from build123d import *

# Parameters (mm, degrees)
BOSS_EXTRUDE1_DEPTH = 10
BOSS_EXTRUDE2_DEPTH = 10
FILLET1_R           = 1


with BuildPart() as part:
    # Sketch1 → Boss-Extrude1 (new body)
    with BuildSketch(Plane(origin=(0, 0, 0), x_dir=(1, 0, 0), z_dir=(0, 1, 0))):
        Polygon((0, 0), (2, 0.535898385), (2, 23.5), (0, 23.5), align=None)
    extrude(amount=BOSS_EXTRUDE1_DEPTH)

    # Sketch3 → Boss-Extrude2 (add)
    with BuildSketch(Plane.XZ):
        Polygon((0, 0), (115.911099155, -31.058285412), (115.285791267, -32.958019616), (0, -2), align=None)
    extrude(amount=-BOSS_EXTRUDE2_DEPTH)

    # Fillet1
    fillet1_edges = [part.edges().sort_by_distance(p)[0] for p in [
        (2, 5, -2.537065657),
        (0, 5, 0),
    ]]
    fillet(fillet1_edges, radius=FILLET1_R)


solid = part.part
Geometry check sheet. Reference: the model listing, model coordinates, mm. A direction names the side the tool comes from. Coordinates: 2 decimals unless noted, no trailing zeros. Order: outer loops, then holes, each group sorted by start corner. A loop starts at its lowest first (then second) coordinate and runs counter-clockwise, first axis right, second up. Notation, with made-up numbers: (68, 14) -> (123, 14) arc R35 cw to (123, 51) -> close; hole circle Ø10 at (51, -10). An arc over 180 degrees is marked (long way). Use a Markdown table: item, result. Add a question column.
1. Go/stop test with flat-tipped pins: pin 1 Ø5 at (x, y) = (69, 8.5) entering from -Z; pin 2 Ø0.6 at (x, y) = (1, 2.5) entering from -Z; pin 3 Ø1 at (x, y) = (26.5, 4.5) entering from -Z. Record where each tip stops, or that it passes through.
2. Cross-section at C-C (z = -10). Enter the section's corners in (x, y), and give its area (3 significant figures).
3. Set-up check for faces 1 (the face through (0, 5, -13)), 2 (the face through (2, 5, -14)): record each of +Z, -Z, +X, -X, +Y, -Y from which the full face is reachable in a straight line by a thin tool's end or side.
4. Mould release check, pull along X, two halves, no side actions. Record for faces 3 (the face through (115.6, 4.9, -32)), 4 (the face through (1, 5, -23.5)), 5 (the face through (60.06, 4.93, -18.13)): pulls with the +X half, pulls with the -X half, needs draft (parallel to the pull), parting line crosses it, or undercut.
5. Cross-section at D-D (x = 47.5). Enter the section's corners in (y, z).
6. Material ranges on L1, parallel to Z at x = 7.5, y = 1.25; L2, parallel to Z at x = 107.5, y = 8.25, recorded low to high.
7. Cross-section at B-B (y = 3.25). Enter the section's corners in (x, z).
8. Cross-section at A-A (z = -18). Enter the section's corners in (x, y), and give its area (3 significant figures).
Filled sheet:
| question | item | result |
|---|---|---|
| 1 | pin 1 | z = -21.2 |
| 1 | pin 2 | z = -23.5 |
| 1 | pin 3 | z = -9.25 |
| 2 | outline | (0, 0) -> (2, 0) -> (2, 10) -> (0, 10) -> close; (29.79, 0) -> (37.32, 0) -> (37.32, 10) -> (29.79, 10) -> close |
| 2 | area | 95.3 mm2 |
| 3 | face 1 | +Z, -Z, -X, +Y, -Y |
| 3 | face 2 | -Z, +Y, -Y |
| 4 | face 3 | pulls with the +X half |
| 4 | face 4 | needs draft |
| 4 | face 5 | undercut |
| 5 | outline | (0, -14.76) -> (10, -14.76) -> (10, -12.73) -> (0, -12.73) -> close |
| 6 | L1 | -4.01 to -2.01 |
| 6 | L2 | -30.87 to -28.8 |
| 7 | outline | (0, -23.5) -> (2, -23.5) -> (2, -3.84) arc R1 cw to (3.26, -2.88) -> (115.29, -32.96) -> (115.91, -31.06) -> (1.26, -0.34) arc R1 ccw to (0, -1.3) -> close |
| 8 | outline | (0, 0) -> (2, 0) -> (2, 10) -> (0, 10) -> close; (59.58, 0) -> (67.18, 0) -> (67.18, 10) -> (59.58, 10) -> close |
| 8 | area | 95.9 mm2 |
